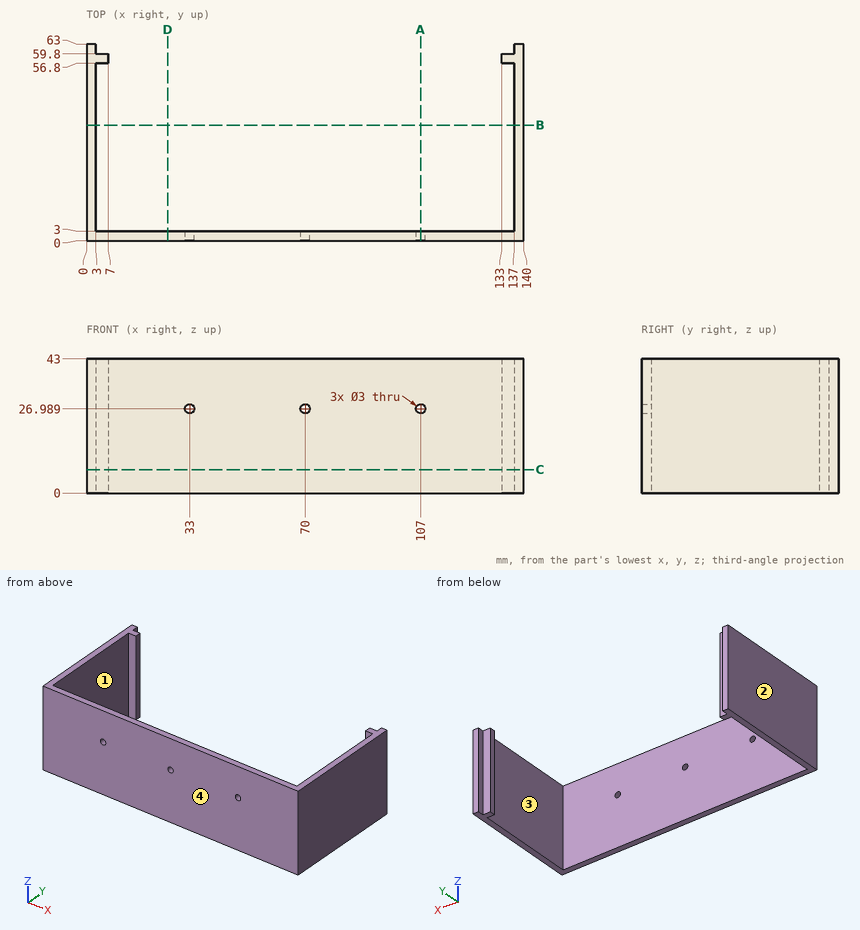
Geometry check sheet. Reference: drawing and pictorial views, mm from the part's lowest x, y, z. Round coordinates to 2 decimals unless told otherwise and drop trailing zeros. Write each loop counter-clockwise with the first axis right and the second up, starting at its lowest first coordinate (ties: lowest second). Pieces come first, ordered by that corner, then holes. Notation, with made-up numbers: (-19.75, 61.25) -> (-14.75, 61.25) arc R21 ccw to (-14.75, 67.25) -> close; hole circle Ø8 at (-29.5, 41.5). An arc over 180 degrees is marked (long way). One line per question, with ' | ' between items. Start each with the question number.
1. Sectioned sample at C-C, the plane z = 7.5. Record the cut outline in (x, y), then the cut area to 3 significant figures.
2. Scan lines: line 1 along X through (y, z) = (20, 27.5); line 2 along Z through (x, y) = (33, 2.2); line 3 along Y through (x, z) = (133.5, 9.5). Record each from-to range of solid material in increasing order. Write a range as from..to.
3. Sectioned sample at A-A, the plane x = 107. Record the cut outline in (y, z).
4. Depth check by flat-ended pin: pin 1 (1.6 mm diameter, centred on y = 62, z = 15.5, fed in from -X); pin 2 (3.5 mm diameter, centred on x = 107, z = 26.99, fed in from +Y); pin 3 (12 mm diameter, centred on x = 104, y = 12, fed in from -Z); pin 4 (2 mm diameter, centred on x = 135, z = 30.5, fed in from +Y). Enter the tip coordinate at first touch or a pass-through.
5. Sectioned sample at D-D, the plane x = 26. Record the cut outline in (y, z), then the cut area to 3 significant figures.
6. Release check for a two-part mould opening along X. For the marked faces 1, 2, 3 and 4 record: +X half, -X half, draft (parallel to the pull), parting line (faces both ways), or undercut.
7. Sectioned sample at B-B, the plane y = 37. Record the cut outline in (x, z), then the cut area to 3 significant figures.
Taken from the geometry:
1) outline: (0, 0) -> (140, 0) -> (140, 63) -> (137, 63) -> (137, 59.8) -> (133, 59.8) -> (133, 56.8) -> (137, 56.8) -> (137, 3) -> (3, 3) -> (3, 56.8) -> (7, 56.8) -> (7, 59.8) -> (3, 59.8) -> (3, 63) -> (0, 63) -> close | area: 804 mm^2
2) line 1: x = 0..3, 137..140 | line 2: z = 0..25.49, 28.49..43 | line 3: y = 0..3, 56.8..59.8
3) outline: (0, 0) -> (3, 0) -> (3, 25.49) -> (0, 25.49) -> close; (0, 28.49) -> (3, 28.49) -> (3, 43) -> (0, 43) -> close
4) pin 1: stops at x = 0 | pin 2: stops at y = 3 | pin 3: passes through | pin 4: stops at y = 59.8
5) outline: (0, 0) -> (3, 0) -> (3, 43) -> (0, 43) -> close | area: 129 mm^2
6) face 1: undercut | face 2: -X half | face 3: undercut | face 4: draft
7) outline: (0, 0) -> (3, 0) -> (3, 43) -> (0, 43) -> close; (137, 0) -> (140, 0) -> (140, 43) -> (137, 43) -> close | area: 258 mm^2
